```python
from build123d import *

# Parameters (mm, degrees)
ESQUISSE1_W             = 25
ESQUISSE1_H             = 40
BOSS_EXTRU_1_DEPTH      = 3.175
ENL_V_MAT_EXTRU_1_REACH = 26.425
ESQUISSE2_R             = 1.83
CONG_1_R                = 2


with BuildPart() as part:
    # Esquisse1 → Boss.-Extru.1 (new, symmetric)
    with BuildSketch(Plane.XY):
        Rectangle(ESQUISSE1_W, ESQUISSE1_H)
    extrude(amount=BOSS_EXTRU_1_DEPTH, both=True)

    # Esquisse2 → Enlèv. mat.-Extru.1 (cut, up to next)
    with BuildSketch(Plane.XY.offset(3.175), mode=Mode.PRIVATE) as enl_v_mat_extru_1_sk1:
        with Locations((-8.5, 16)):
            Circle(ESQUISSE2_R)
    enl_v_mat_extru_1_tool1 = extrude(enl_v_mat_extru_1_sk1.sketch, amount=-ENL_V_MAT_EXTRU_1_REACH, mode=Mode.PRIVATE) & part.part
    # Esquisse2 → Enlèv. mat.-Extru.1 (cut, up to next)
    with BuildSketch(Plane.XY.offset(3.175), mode=Mode.PRIVATE) as enl_v_mat_extru_1_sk2:
        with Locations((8.5, 16)):
            Circle(ESQUISSE2_R)
    enl_v_mat_extru_1_tool2 = extrude(enl_v_mat_extru_1_sk2.sketch, amount=-ENL_V_MAT_EXTRU_1_REACH, mode=Mode.PRIVATE) & part.part
    # Esquisse2 → Enlèv. mat.-Extru.1 (cut, up to next)
    with BuildSketch(Plane.XY.offset(3.175), mode=Mode.PRIVATE) as enl_v_mat_extru_1_sk3:
        with Locations((8.5, -16)):
            Circle(ESQUISSE2_R)
    enl_v_mat_extru_1_tool3 = extrude(enl_v_mat_extru_1_sk3.sketch, amount=-ENL_V_MAT_EXTRU_1_REACH, mode=Mode.PRIVATE) & part.part
    # Esquisse2 → Enlèv. mat.-Extru.1 (cut, up to next)
    with BuildSketch(Plane.XY.offset(3.175), mode=Mode.PRIVATE) as enl_v_mat_extru_1_sk4:
        with Locations((-8.5, -16)):
            Circle(ESQUISSE2_R)
    enl_v_mat_extru_1_tool4 = extrude(enl_v_mat_extru_1_sk4.sketch, amount=-ENL_V_MAT_EXTRU_1_REACH, mode=Mode.PRIVATE) & part.part
    add(enl_v_mat_extru_1_tool1.solids().sort_by_distance((-8.5, 16, 3.175))[0], mode=Mode.SUBTRACT)
    add(enl_v_mat_extru_1_tool2.solids().sort_by_distance((8.5, 16, 3.175))[0], mode=Mode.SUBTRACT)
    add(enl_v_mat_extru_1_tool3.solids().sort_by_distance((8.5, -16, 3.175))[0], mode=Mode.SUBTRACT)
    add(enl_v_mat_extru_1_tool4.solids().sort_by_distance((-8.5, -16, 3.175))[0], mode=Mode.SUBTRACT)

    # Congé1
    cong_1_edges = [part.edges().sort_by_distance(p)[0] for p in [
        (-12.5, 20, 0),
        (12.5, 20, 0),
        (12.5, -20, 0),
        (-12.5, -20, 0),
    ]]
    fillet(cong_1_edges, radius=CONG_1_R)


solid = part.part
```
Design review of the part built by this model. Coordinates are the model's own, in mm. Coordinates: 2 decimals unless noted, no trailing zeros. Loops run counter-clockwise (first coordinate to the right, second up) from the corner with the lowest first, then second, coordinate; pieces in that order, holes last. Notation, with made-up numbers: (2, 66.5) -> (43, 66.5) arc R24 ccw to (43, 89.5) -> close; hole circle Ø7 at (56, 64). An arc over 180 degrees is marked (long way). Answer as a JSON object with one key per item and string values.
Q1. Take a section at B-B on x = 7.5. Give the boundary of the cut face in (y, z) (3 decimals), plus the area to 3 significant figures.
Answer block:
{"outline": "(-20, -3.175) -> (-17.533, -3.175) -> (-17.533, 3.175) -> (-20, 3.175) -> close; (-14.467, -3.175) -> (14.467, -3.175) -> (14.467, 3.175) -> (-14.467, 3.175) -> close; (17.533, -3.175) -> (20, -3.175) -> (20, 3.175) -> (17.533, 3.175) -> close", "area": "215 mm^2"}
Q2. The part is to be moulded in two halves that separate along Y. For faces 1 (the cylindrical face through (-8.738, -14.186, 0.044)), 2 (the cylindrical face through (11.9, 19.43, -0.04)), 3 (the cylindrical face through (-11.93, -19.4, 0.04)), say which applies: +Y half, -Y half, draft (parallel to the pull), parting line (faces both ways), or undercut.
Answer block:
{"face 1": "undercut", "face 2": "+Y half", "face 3": "-Y half"}
Q3. To check wall thickness, follow L1, parallel to Y at x = -8.5, z = -1.5; L2, parallel to X at y = 17.5, z = -2; L3, parallel to Y at x = 7.75, z = 1. State the ranges of each line that lie inside material, in increasing order.
Answer block:
{"L1": "y = -20 to -17.83, -14.17 to 14.17, 17.83 to 20", "L2": "x = -12.5 to -9.55, -7.45 to 7.45, 9.55 to 12.5", "L3": "y = -20 to -17.67, -14.33 to 14.33, 17.67 to 20"}
Q4. Take a section at C-C on z = 0.75. Give the boundary of the cut face in (x, y), plus the area to 3 significant figures.
Answer block:
{"outline": "(-12.5, -18) arc R2 ccw to (-10.5, -20) -> (10.5, -20) arc R2 ccw to (12.5, -18) -> (12.5, 18) arc R2 ccw to (10.5, 20) -> (-10.5, 20) arc R2 ccw to (-12.5, 18) -> close; hole circle Ø3.66 at (-8.5, -16); hole circle Ø3.66 at (-8.5, 16); hole circle Ø3.66 at (8.5, -16); hole circle Ø3.66 at (8.5, 16)", "area": "954 mm^2"}
Q5. Take a section at A-A on y = -16. Give the boundary of the cut face in (x, z) (3 decimals).
Answer block:
{"outline": "(-12.5, -3.175) -> (-10.33, -3.175) -> (-10.33, 3.175) -> (-12.5, 3.175) -> close; (-6.67, -3.175) -> (6.67, -3.175) -> (6.67, 3.175) -> (-6.67, 3.175) -> close; (10.33, -3.175) -> (12.5, -3.175) -> (12.5, 3.175) -> (10.33, 3.175) -> close"}
